from build123d import *

# Parameters (mm, degrees)
SKETCH1_R           = 6
BOSS_EXTRUDE1_DEPTH = 1
SKETCH2_R           = 4.725
BOSS_EXTRUDE2_DEPTH = 2.7
CUT_EXTRUDE1_DEPTH  = 10.256889326


with BuildPart() as part:
    # Sketch1 → Boss-Extrude1 (new body)
    with BuildSketch(Plane(origin=(0, 0, 0), x_dir=(1, 0, 0), z_dir=(0, 1, 0))):
        with Locations(Location((0, 0, 0), (0, 0, 270))):
            Circle(SKETCH1_R)
    extrude(amount=BOSS_EXTRUDE1_DEPTH)

    # Sketch2 → Boss-Extrude2 (add)
    with BuildSketch(Plane(origin=(0, 1, 0), x_dir=(1, 0, 0), z_dir=(0, 1, 0))):
        with Locations(Location((0, 0, 0), (0, 0, 90))):
            Circle(SKETCH2_R)
    extrude(amount=BOSS_EXTRUDE2_DEPTH)

    # Sketch3 → Cut-Extrude1 (cut, through all)
    with BuildSketch(Plane(origin=(0, 3.7, 0), x_dir=(1, 0, 0), z_dir=(0, 1, 0))):
        with BuildLine():
            Line((2.475, 2.294558781), (2.475, -2.294558781))
            ThreePointArc((2.475, -2.294558781), (-3.375, 0), (2.475, 2.294558781))
        make_face()
    extrude(amount=-CUT_EXTRUDE1_DEPTH, mode=Mode.SUBTRACT)


solid = part.part
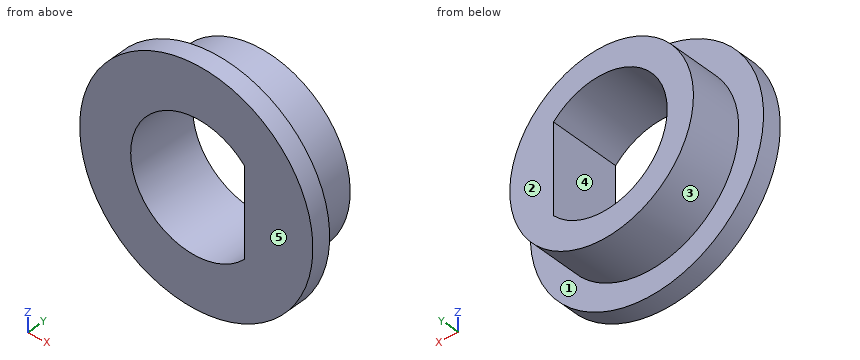
Check sheet for the modelled part. Datum: model origin and axes. Units: mm. Face numbers are marked on the shaded views. A direction names the side the tool comes from. Round coordinates to 2 decimals unless told otherwise and drop trailing zeros. Order: outer loops, then holes, each group sorted by start corner. A loop starts at its lowest first (then second) coordinate and runs counter-clockwise, first axis right, second up.
(1) Draft check along Z on the marked faces 3, 4 and 5. Enter one of: pulls with the +Z half, pulls with the -Z half, needs draft (parallel to the pull), parting line crosses it, or undercut.
(2) Cross-section at D-D, the plane x = -4.5. Enter the section's corners in (y, z), and give its area (3 significant figures).
(3) Cross-section at C-C, the plane y = 2.6. Enter the section's corners in (x, z) (3 decimals), and give its area (3 significant figures).
(4) Cross-section at A-A, the plane z = 0. Enter the section's corners in (x, y) (3 decimals).
(5) Scan lines: probe 1 along X at (y, z) = (2.75, 0) (3 decimals); probe 2 along X at (y, z) = (1.8, -3); probe 3 along Y at (x, z) = (3, 4.5). Record each from-to range of solid material in increasing order.
(6) Access from +Z, -Z, +X, -X, +Y, -Y to the whole of each face (thin tool, end or side, straight path). Record for the marked faces 1 and 2.
(7) Go/stop test with flat-tipped pins: P1, Ø3, axis at x = -1.5, z = 1, coming from the -Y side; P2, Ø1.5, axis at y = 2, z = -3.5, coming from the -X side; P3, Ø1, axis at x = 4.5, z = 4, coming from the +Y side; P4, Ø1, axis at x = 2, y = 2, coming from the +Z side. Record where each tip stops, or that it passes through.
(8) Cross-section at B-B, the plane x = 0. Enter the section's corners in (y, z) (3 decimals).
Check sheet entries:
1. face 3: parting line crosses it
1. face 4: undercut
1. face 5: needs draft
2. outline: (0, -3.97) - (1, -3.97) - (1, -1.44) - (3.7, -1.44) - (3.7, 1.44) - (1, 1.44) - (1, 3.97) - (0, 3.97) - close
2. area: 15.7 mm2
3. outline: circle Ø9.45 at (0, 0); hole (2.475, -2.295) - (2.475, 2.295) arc R3.375 ccw (long way) to start
3. area: 37.2 mm2
4. outline: (-6, 0) - (-3.375, 0) - (-3.375, 3.7) - (-4.725, 3.7) - (-4.725, 1) - (-6, 1) - close; (2.475, 0) - (6, 0) - (6, 1) - (4.725, 1) - (4.725, 3.7) - (2.475, 3.7) - close
5. probe 1: x = -4.725 to -3.375, 2.475 to 4.725
5. probe 2: x = -3.65 to -1.55, 1.55 to 3.65
5. probe 3: y = 0 to 1
6. face 1: +Y
6. face 2: +Z, -Z, +X, -X, +Y
7. P1: passes through
7. P2: stops at x = -3.84
7. P3: stops at y = 1
7. P4: stops at z = 4.48
8. outline: (0, -6) - (1, -6) - (1, -4.725) - (3.7, -4.725) - (3.7, -3.375) - (0, -3.375) - close; (0, 3.375) - (3.7, 3.375) - (3.7, 4.725) - (1, 4.725) - (1, 6) - (0, 6) - close
